Design review of the part built by this model. Coordinates are the model's own, in mm. Give positions to 0.01 mm unless a question says otherwise; leave off trailing zeros. Write each loop counter-clockwise with the first axis right and the second up, starting at its lowest first coordinate (ties: lowest second). Pieces come first, ordered by that corner, then holes. Notation, with made-up numbers: (2, 36.5) -> (32, 36.5) arc R21 cw to (32, 75.5) -> close; hole circle Ø8 at (-1.5, 36.25). An arc over 180 degrees is marked (long way). Answer as a JSON object with one key per item and string values.
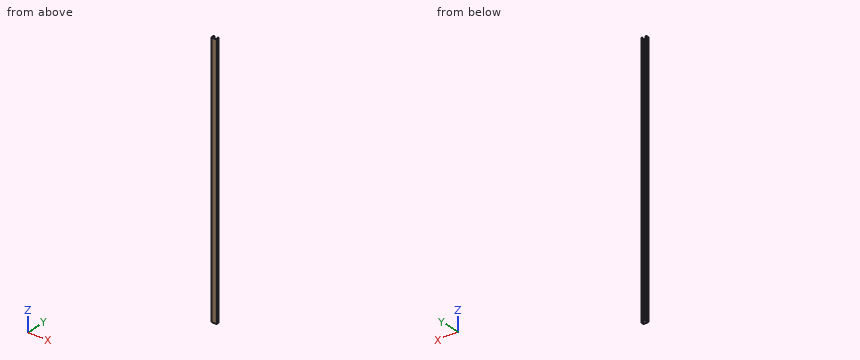
Autodesk Inventor part; units mm, degrees
ref_plane "Work Plane1" through (0, 0, 0) normal (0, 0, 1) x (1, 0, 0)
ref_plane "YZ Plane" through (0, 0, 0) normal (1, 0, 0) x (0, 1, 0)
ref_plane "XZ Plane" through (0, 0, 0) normal (0, 1, 0) x (-1, 0, 0)
ref_plane "Work Plane1" through (0, 0, 0) normal (0, 0, 1) x (1, 0, 0)
sketch "Sketch1" plane through (0, 0, 0) normal (0, 0, 1) x (1, 0, 0)
  arc A0 (-113.2188, 0) -> (-109.7581, 3.4607) centre (-113.2188, 3.4607) ccw
  line L0 (-109.7581, 17.1767) -> (-109.7581, 3.4607)
  arc A1 (-109.7581, 17.1767) -> (-114.8063, 22.225) centre (-114.8063, 17.1767) ccw
  line L1 (-115.8223, 22.225) -> (-114.8063, 22.225)
  arc A2 (-115.8223, 22.225) -> (-119.2831, 18.7642) centre (-115.8223, 18.7642) ccw
  line L2 (-119.2831, 16.4211) -> (-119.2831, 18.7642)
  arc A3 (-119.2831, 16.4211) -> (-116.6161, 16.4211) centre (-117.9496, 16.4211) ccw
  line L3 (-116.6161, 18.7642) -> (-116.6161, 16.4211)
  arc A4 (-115.8223, 19.558) -> (-116.6161, 18.7642) centre (-115.8223, 18.7642) ccw
  line L4 (-114.8063, 19.558) -> (-115.8223, 19.558)
  arc A5 (-112.4251, 17.1767) -> (-114.8063, 19.558) centre (-114.8063, 17.1767) ccw
  line L5 (-112.4251, 3.4607) -> (-112.4251, 17.1767)
  arc A6 (-113.2188, 2.667) -> (-112.4251, 3.4607) centre (-113.2188, 3.4607) ccw
  line L6 (-147.5723, 2.667) -> (-113.2188, 2.667)
  arc A7 (-148.3661, 3.4607) -> (-147.5723, 2.667) centre (-147.5723, 3.4607) ccw
  line L7 (-148.3661, 17.1767) -> (-148.3661, 3.4607)
  arc A8 (-145.9848, 19.558) -> (-148.3661, 17.1767) centre (-145.9848, 17.1767) ccw
  line L8 (-144.9688, 19.558) -> (-145.9848, 19.558)
  arc A9 (-144.1751, 18.7642) -> (-144.9688, 19.558) centre (-144.9688, 18.7642) ccw
  line L9 (-144.1751, 16.4211) -> (-144.1751, 18.7642)
  arc A10 (-144.1751, 16.4211) -> (-141.5081, 16.4211) centre (-142.8416, 16.4211) ccw
  line L10 (-141.5081, 18.7642) -> (-141.5081, 16.4211)
  arc A11 (-141.5081, 18.7642) -> (-144.9688, 22.225) centre (-144.9688, 18.7642) ccw
  line L11 (-145.9848, 22.225) -> (-144.9688, 22.225)
  arc A12 (-145.9848, 22.225) -> (-151.0331, 17.1767) centre (-145.9848, 17.1767) ccw
  line L12 (-151.0331, 3.4607) -> (-151.0331, 17.1767)
  arc A13 (-151.0331, 3.4607) -> (-147.5723, 0) centre (-147.5723, 3.4607) ccw
  line L13 (-113.2188, 0) -> (-147.5723, 0)
  point P0 (0, 0)
extrude "Extrusion1" add sketch "Sketch1" along normal blind 1905
properties part number "Unistrut 75"
(1) We need section B-B, the plane z = 1133. State the section outline as (x, y) points (1 decimal), then the cut area to 3 significant figures.
Here are the results:
{"outline": "(-151, 3.5) arc R3.5 ccw to (-147.6, 0) -> (-113.2, 0) arc R3.5 ccw to (-109.8, 3.5) -> (-109.8, 17.2) arc R5 ccw to (-114.8, 22.2) -> (-115.8, 22.2) arc R3.5 ccw to (-119.3, 18.8) -> (-119.3, 16.4) arc R1.3 ccw to (-116.6, 16.4) -> (-116.6, 18.8) arc R0.8 cw to (-115.8, 19.6) -> (-114.8, 19.6) arc R2.4 cw to (-112.4, 17.2) -> (-112.4, 3.5) arc R0.8 cw to (-113.2, 2.7) -> (-147.6, 2.7) arc R0.8 cw to (-148.4, 3.5) -> (-148.4, 17.2) arc R2.4 cw to (-146, 19.6) -> (-145, 19.6) arc R0.8 cw to (-144.2, 18.8) -> (-144.2, 16.4) arc R1.3 ccw to (-141.5, 16.4) -> (-141.5, 18.8) arc R3.5 ccw to (-145, 22.2) -> (-146, 22.2) arc R5 ccw to (-151, 17.2) -> close", "area": "255 mm²"}
(2) For line 1 along X through (y, z) = (16.5, 261.5); line 2 along X through (y, z) = (14, 549.5); line 3 along Y through (x, z) = (-146.5, 1161), list the stretches that pass through material, from the lowest coordinate up.
Here are the results:
{"line 1": "x = -151.03 to -148.37, -144.18 to -141.51, -119.28 to -116.62, -112.43 to -109.76", "line 2": "x = -151.03 to -148.37, -112.43 to -109.76", "line 3": "y = 0 to 2.67, 19.5 to 22.2"}
(3) Clearance check with flat-ended pins moving along their axes: pin 1 (1.5 mm diameter, centred on y = 2.5, z = 1675.5, fed in from +X); pin 2 (6 mm diameter, centred on x = -142, y = 10, fed in from +Z). State where each tip first meets the part, or that it passes through.
Here are the results:
{"pin 1": "stops at x = -109.76", "pin 2": "passes through"}
(4) We need section A-A, the plane y = 8.25. State the section outline as (x, z) points, then the cut area to 3 significant figures.
Here are the results:
{"outline": "(-151.03, 0) -> (-148.37, 0) -> (-148.37, 1905) -> (-151.03, 1905) -> close; (-112.43, 0) -> (-109.76, 0) -> (-109.76, 1905) -> (-112.43, 1905) -> close", "area": "10,200 mm²"}
(5) We need section C-C, the plane x = -128.5. State the section outline as (y, z) points, then the cut area to 3 significant figures.
Here are the results:
{"outline": "(0, 0) -> (2.67, 0) -> (2.67, 1905) -> (0, 1905) -> close", "area": "5,080 mm²"}
